Can you work these out from the model? Positions are in its coordinate system, mm. A direction names the side the tool comes from. Give positions to 0.01 mm unless a question says otherwise; leave off trailing zeros. Loops run counter-clockwise (first coordinate to the right, second up) from the corner with the lowest first, then second, coordinate; pieces in that order, holes last. Notation, with made-up numbers: (-37, 28.25) -> (-18, 28.25) arc R28 ccw to (-18, 58.25) -> close; hole circle Ø6 at (88.5, -10). An arc over 180 degrees is marked (long way). Use CSV: the item, a comma, the result in double quotes.
from build123d import *

# Parameters (mm, degrees)
SKETCH1_R           = 30
SKETCH1_R_2         = 15
BOSS_EXTRUDE1_DEPTH = 20
BOSS_EXTRUDE2_DEPTH = 20
SKETCH3_R           = 1
CUT_EXTRUDE1_DEPTH  = 20
SKETCH4_R           = 7.5
BOSS_EXTRUDE3_DEPTH = 20


with BuildPart() as part:
    # Sketch1 → Boss-Extrude1 (new body)
    with BuildSketch(Plane(origin=(0, 0, 0), x_dir=(1, 0, 0), z_dir=(0, 1, 0))):
        Circle(SKETCH1_R)
        with BuildLine():
            ThreePointArc((-2.5, -24.874685928), (-25, 0), (-2.5, 24.874685928))
            Line((-2.5, 24.874685928), (-2.5, 19.843134833))
            ThreePointArc((-2.5, 19.843134833), (0, -20), (2.5, 19.843134833))
            Line((2.5, 19.843134833), (2.5, 24.874685928))
            ThreePointArc((2.5, 24.874685928), (25, 0), (2.5, -24.874685928))
            Line((2.5, -24.874685928), (2.5, -26.5))
            ThreePointArc((2.5, -26.5), (2.207106781, -27.207106781), (1.5, -27.5))
            Line((1.5, -27.5), (-1.5, -27.5))
            ThreePointArc((-1.5, -27.5), (-2.207106781, -27.207106781), (-2.5, -26.5))
            Line((-2.5, -26.5), (-2.5, -24.874685928))
        make_face(mode=Mode.SUBTRACT)
        Circle(SKETCH1_R_2, mode=Mode.SUBTRACT)
    extrude(amount=BOSS_EXTRUDE1_DEPTH)

    # Sketch2 → Boss-Extrude2 (add)
    with BuildSketch(Plane(origin=(0, 20, 0), x_dir=(1, 0, 0), z_dir=(0, 1, 0))):
        with BuildLine():
            Line((27.271780287, 10), (27.271780287, -10))
            ThreePointArc((27.271780287, -10), (37.271780287, 0), (27.271780287, 10))
        make_face()
    extrude(amount=-BOSS_EXTRUDE2_DEPTH)

    # Sketch3 → Cut-Extrude1 (cut)
    with BuildSketch(Plane(origin=(0, 20, 0), x_dir=(1, 0, 0), z_dir=(0, 1, 0))):
        with Locations((33, 0)):
            Circle(SKETCH3_R)
    extrude(amount=-CUT_EXTRUDE1_DEPTH, mode=Mode.SUBTRACT)

    # Sketch4 → Boss-Extrude3 (add)
    with BuildSketch(Plane(origin=(0, 0, 0), x_dir=(1, 0, 0), z_dir=(0, 1, 0))):
        with BuildLine():
            Line((-2.5, 19.843134833), (2.5, 19.843134833))
            Line((2.5, 19.843134833), (2.5, 12.247448714))
            ThreePointArc((2.5, 12.247448714), (8.838834765, 8.838834765), (12.247448714, 2.5))
            Line((12.247448714, 2.5), (16.124945742, 2.5))
            Line((16.124945742, 2.5), (16.124945742, -2.5))
            Line((16.124945742, -2.5), (12.247448714, -2.5))
            ThreePointArc((12.247448714, -2.5), (8.838834765, -8.838834765), (2.5, -12.247448714))
            Line((2.5, -12.247448714), (2.5, -17.575657714))
            Line((2.5, -17.575657714), (-2.5, -17.575657714))
            Line((-2.5, -17.575657714), (-2.5, -12.247448714))
            ThreePointArc((-2.5, -12.247448714), (-8.838834765, -8.838834765), (-12.247448714, -2.5))
            Line((-12.247448714, -2.5), (-16.958645249, -2.5))
            Line((-16.958645249, -2.5), (-16.958645249, 2.5))
            Line((-16.958645249, 2.5), (-12.247448714, 2.5))
            ThreePointArc((-12.247448714, 2.5), (-8.838834765, 8.838834765), (-2.5, 12.247448714))
            Line((-2.5, 12.247448714), (-2.5, 19.843134833))
        make_face()
        Circle(SKETCH4_R, mode=Mode.SUBTRACT)
    extrude(amount=BOSS_EXTRUDE3_DEPTH)


solid = part.part
(1) If I drill on L1, parallel to X at y = 11.5, z = 0; L2, parallel to X at y = 1, z = -17.5; L3, parallel to X at y = 15.5, z = -8, over which ranges is the centre line in solid material (lowest first)? Write a range as from..to.
Answer sheet:
L1,"x = -30..-25, -20..-7.5, 7.5..20, 25..32, 34..37.27"
L2,"x = -24.37..-17.85, -9.68..9.68, 17.85..24.37"
L3,"x = -28.91..-23.69, -18.33..-12.69, -9.6..9.6, 12.69..18.33, 23.69..33.27"
(2) If we section it at D-D, the plane x = 24: Write out the boundary of the cut face in (y, z), then the cut area to 3 significant figures.
Answer sheet:
outline,"(0, -18) -> (20, -18) -> (20, -7) -> (0, -7) -> close; (0, 7) -> (20, 7) -> (20, 18) -> (0, 18) -> close"
area,"440 mm2"
(3) We'd pull the mould along Z, two halves only. Please class faces 1 (the face through (37.27, 10.14, 0.21)), 2 (the face through (11, 20, 0)), 3 (the face through (14, 10, -2.5)): released by +Z, released by -Z, zero draft, split by the parting line, or undercut.
Answer sheet:
face 1,"split by the parting line"
face 2,"zero draft"
face 3,"undercut"
(4) Which directions (+Z, -Z, +X, -X, +Y, -Y) give clear straight access to the entire face, cutting with the end or side of a thin tool? Please do faces 4 (the face through (-2.5, 10, -22)), 5 (the face through (11, 0, 0)).
Answer sheet:
face 4,"+Y, -Y"
face 5,"+Z, -Z, +X, -X, -Y"
(5) If we section it at B-B, the plane x = 0: Write out the boundary of the cut face in (y, z), then the cut area to 3 significant figures.
Answer sheet:
outline,"(0, -30) -> (20, -30) -> (20, -7.5) -> (0, -7.5) -> close; (0, 7.5) -> (20, 7.5) -> (20, 20) -> (0, 20) -> close; (0, 27.5) -> (20, 27.5) -> (20, 30) -> (0, 30) -> close"
area,"750 mm2"
(6) If we section it at C-C, the plane z = -24: Write out the boundary of the cut face in (x, y).
Answer sheet:
outline,"(-18, 0) -> (-7, 0) -> (-7, 20) -> (-18, 20) -> close; (-2.5, 0) -> (2.5, 0) -> (2.5, 20) -> (-2.5, 20) -> close; (7, 0) -> (18, 0) -> (18, 20) -> (7, 20) -> close"
(7) If we section it at A-A, the plane z = 0: Write out the boundary of the cut face in (x, y), then the cut area to 3 significant figures.
Answer sheet:
outline,"(-30, 0) -> (-25, 0) -> (-25, 20) -> (-30, 20) -> close; (-20, 0) -> (-7.5, 0) -> (-7.5, 20) -> (-20, 20) -> close; (7.5, 0) -> (20, 0) -> (20, 20) -> (7.5, 20) -> close; (25, 0) -> (32, 0) -> (32, 20) -> (25, 20) -> close; (34, 0) -> (37.27, 0) -> (37.27, 20) -> (34, 20) -> close"
area,"805 mm2"
(8) Will these pins go through, and if not, where does the flat tip stop? pin 1 Ø4 at (y, z) = (14, -22.5) entering from -X; pin 2 Ø1.5 at (x, y) = (-2, 9) entering from +Z; pin 3 Ø3 at (y, z) = (7.5, 14) entering from -X; pin 4 Ø4 at (x, z) = (-14, -18) entering from +Y.
Answer sheet:
pin 1,"stops at x = -21.9"
pin 2,"stops at z = 29.97"
pin 3,"stops at x = -27.27"
pin 4,"passes through"
